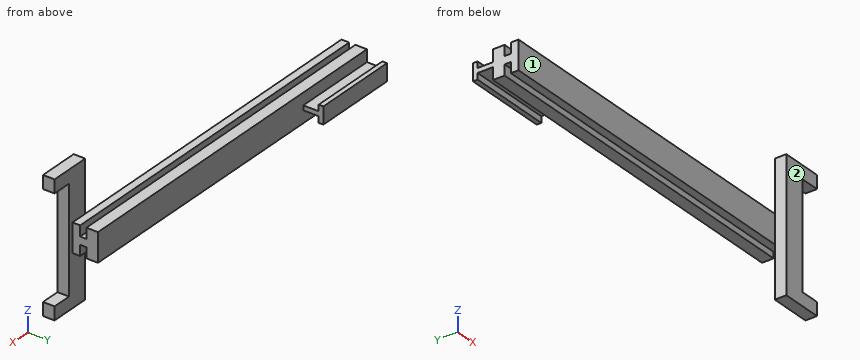
Autodesk Inventor part; units mm, degrees
ref_plane "YZ Plane" through (0, 0, 0) normal (1, 0, 0) x (0, 1, 0)
ref_plane "XZ Plane" through (0, 0, 0) normal (0, 1, 0) x (-1, 0, 0)
ref_plane "XY Plane" through (0, 0, 0) normal (0, 0, 1) x (1, 0, 0)
sketch "Esboço1" plane through (0, 0, 0) normal (0, 1, 0) x (-1, 0, 0)
  line L0 (0, 0) -> (0, -18.5)
  line L1 (0, 0) -> (232.5, 0)
  line L2 (232.5, 0) -> (232.5, -18.5)
  line L3 (232.5, -18.5) -> (0, -18.5)
  dimension "d0" = 18.5
  dimension "d1" = 232.5
extrude "Extrusão1" add sketch "Esboço1" along normal blind 5
sketch "Esboço2" plane through (0, 5, 0) normal (0, 1, 0) x (1, 0, 0)
  line L0 (0, 0) -> (0, 9.25)
  line L1 (0, 0) -> (0, 18.5)
  line L2 (0, 9.25) -> (0, 11.75)
  line L3 (0, 11.75) -> (0, 6.75)
  line L4 (0, 6.75) -> (-232.5, 6.75)
  line L5 (-232.5, 18.5) -> (-232.5, 0)
  line L6 (-232.5, 6.75) -> (-232.5, 11.75)
  line L7 (-232.5, 11.75) -> (0, 11.75)
  dimension "d4" = 2.5
  dimension "d5" = 5
extrude "Extrusão2" add sketch "Esboço2" along normal blind 4
sketch "Esboço3" plane through (0, 9, 0) normal (0, 1, 0) x (1, 0, 0)
  line L0 (-232.5, 6.75) -> (0, 6.75)
  line L1 (0, 0) -> (0, 18.5)
  line L2 (0, 6.75) -> (0, 18.5)
  line L3 (0, 18.5) -> (0, 0)
  line L4 (0, 0) -> (-232.5, 0)
  line L5 (0, 18.5) -> (-232.5, 18.5)
  line L6 (-232.5, 18.5) -> (-232.5, 11.75)
  line L7 (-232.5, 0) -> (-232.5, 18.5)
  line L8 (-232.5, 18.5) -> (0, 18.5)
extrude "Extrusão3" add sketch "Esboço3" along normal blind 7.5
sketch "Esboço4" plane through (0, 0, 0) normal (0, -1, 0) x (1, 0, 0)
  line L0 (-232.5, 0) -> (0, 0)
  line L1 (-11, -9.25) -> (-11, -51.75)
  line L2 (-11, -51.75) -> (15.5, -51.75)
  line L3 (15.5, -51.75) -> (15.5, -43.25)
  line L4 (15.5, -43.25) -> (3, -43.25)
  line L5 (-11, -9.25) -> (-11, 33.25)
  line L6 (-11, 33.25) -> (15.5, 33.25)
  line L7 (15.5, 33.25) -> (15.5, 24.75)
  line L8 (15.5, 24.75) -> (3, 24.75)
  line L9 (3, 24.75) -> (3, -43.25)
  dimension "d12" = 42.5
  dimension "d14" = 26.5
  dimension "d15" = 8.5
  dimension "d17" = 42.5
  dimension "d18" = 8.5
extrude "Extrusão4" add sketch "Esboço4" along normal blind 7.5
sketch "Esboço5" plane through (0, 16.5, 0) normal (0, 1, 0) x (1, 0, 0)
  line L0 (0, 18.5) -> (-232.5, 18.5)
  line L1 (-232.5, 18.5) -> (-232.5, 0)
  line L2 (-232.5, 9.25) -> (-232.5, 10.75)
  line L3 (-232.5, 10.75) -> (-232.5, 7.75)
  line L4 (-232.5, 7.75) -> (-177.5, 7.75)
  line L5 (-177.5, 7.75) -> (-177.5, 10.75)
  line L6 (0, 11.75) -> (-232.5, 11.75)
  line L7 (-177.5, 10.75) -> (-232.5, 10.75)
  point P0 (0, 0)
  dimension "d21" = 1.5
  dimension "d22" = 3
  dimension "d23" = 55
  dimension "d24" = 3
extrude "Extrusão5" add sketch "Esboço5" along normal blind 10
sketch "Esboço6" plane through (0, 26.5, 0) normal (0, 1, 0) x (1, 0, 0)
  line L0 (-232.5, 10.75) -> (-232.5, 7.75)
  line L1 (-232.5, 9.25) -> (-232.5, 14.75)
  line L2 (-232.5, 14.75) -> (-232.5, 3.75)
  line L3 (-232.5, 6.75) -> (-232.5, 0)
  line L4 (-232.5, 3.75) -> (-177.5, 3.75)
  line L5 (-177.5, 3.75) -> (-177.5, 14.75)
  line L6 (-177.5, 14.75) -> (-232.5, 14.75)
  line L7 (0, 18.5) -> (-232.5, 18.5)
  point P0 (0, 0)
  dimension "d27" = 5.5
  dimension "d28" = 11
  dimension "d29" = 55
extrude "Extrusão6" add sketch "Esboço6" along normal blind 3
properties part number "trilho sem cremalheira"
The listing builds one solid part. Answer for the finished solid, in the listing's coordinates (mm). Face numbers are marked on the shaded views. A direction names the side the tool comes from. Coordinates: 2 decimals unless noted, no trailing zeros. Loops run counter-clockwise (first coordinate to the right, second up) from the corner with the lowest first, then second, coordinate; pieces in that order, holes last.
1) Find section D-D on z = -28.5. Write down the section's boundary in (x, y).
2) Find the intervals of material crossed by L1, parallel to Y at x = -151, z = -15.5; L2, parallel to X at y = 7, z = -7; L3, parallel to Z at x = -65.5, y = 1.5, in increasing order.
3) Find section C-C on x = -95. Write down the section's boundary in (y, z), then the cut area to 3 significant figures.
4) Flat-ended cylindrical pins translate along their axes: pin 1 Ø1 at (x, y) = (-190.5, 25) entering from -Z; pin 2 Ø2 at (x, y) = (-53, 14) entering from -Z; pin 3 Ø2.5 at (x, y) = (-193.5, 27.5) entering from +Z. Find the tip coordinate at first contact, or state that the pin passes through.
5) Find section A-A on x = -197. Write down the section's boundary in (y, z), then the cut area to 3 significant figures.
6) Find section B-B on y = -3. Write down the section's boundary in (x, z), then the cut area to 3 significant figures.
7) A tool of negligible diameter and unlimited length cuts with its end or side. For the marked faces 1 and 2, from which of +Z, -Z, +X, -X, +Y, -Y can it reach the whole face along a straight path? Write none if from no direction.
Values:
1. outline: (-11, -7.5) - (3, -7.5) - (3, 0) - (-11, 0) - close
2. L1: y = 0 to 5, 9 to 16.5
2. L2: x = -232.5 to 0
2. L3: z = -18.5 to 0
3. outline: (0, -18.5) - (5, -18.5) - (5, -11.75) - (9, -11.75) - (9, -18.5) - (16.5, -18.5) - (16.5, 0) - (9, 0) - (9, -6.75) - (5, -6.75) - (5, 0) - (0, 0) - close
3. area: 251 mm2
4. pin 1: stops at z = -10.75
4. pin 2: stops at z = -18.5
4. pin 3: stops at z = -3.75
5. outline: (0, -18.5) - (5, -18.5) - (5, -11.75) - (9, -11.75) - (9, -18.5) - (16.5, -18.5) - (16.5, -10.75) - (26.5, -10.75) - (26.5, -14.75) - (29.5, -14.75) - (29.5, -3.75) - (26.5, -3.75) - (26.5, -7.75) - (16.5, -7.75) - (16.5, 0) - (9, 0) - (9, -6.75) - (5, -6.75) - (5, 0) - (0, 0) - close
5. area: 314 mm2
6. outline: (-11, -51.75) - (15.5, -51.75) - (15.5, -43.25) - (3, -43.25) - (3, 24.75) - (15.5, 24.75) - (15.5, 33.25) - (-11, 33.25) - close
6. area: 1,400 mm2
7. face 1: +Z, -Z, -X, -Y
7. face 2: +Z, -Z, +X, -X, -Y
